Verification items for the finished model (mm, model axes). Coordinates: 2 decimals unless noted, no trailing zeros. Loops run counter-clockwise (first coordinate to the right, second up) from the corner with the lowest first, then second, coordinate; pieces in that order, holes last. Notation, with made-up numbers: M 28.5,-27.5 L 44.5,-27.5 A35 cw 44.5,8.5 Z; hole C 66.25,3 d8. An arc over 180 degrees is marked long. Write item = value, one per line. Start each with the question number.
```python
from build123d import *

# Parameters (mm, degrees)
ESBO_O1_R                = 1.65
RESSALTO_EXTRUS_O1_DEPTH = 3
FILETE1_R                = 8


with BuildPart() as part:
    # Esboço1 → Ressalto-extrusão1 (new body)
    with BuildSketch(Plane.XY):
        with BuildLine():
            Line((-5.233177242, 16.48), (-11.2845681, 3.348148148))
            ThreePointArc((-11.2845681, 3.348148148), (-11.621333239, 2.490590121), (-11.85726917, 1.6))
            Line((-11.85726917, 1.6), (-7.48080878, 1.6))
            ThreePointArc((-7.48080878, 1.6), (0, 7.65), (7.48080878, 1.6))
            Line((7.48080878, 1.6), (11.85726917, 1.6))
            ThreePointArc((11.85726917, 1.6), (11.621333239, 2.490590121), (11.2845681, 3.348148148))
            Line((11.2845681, 3.348148148), (5.233177242, 16.48))
            Line((5.233177242, 16.48), (-5.233177242, 16.48))
        make_face()
        with Locations((0, 13.5)):
            Circle(ESBO_O1_R, mode=Mode.SUBTRACT)
    extrude(amount=RESSALTO_EXTRUS_O1_DEPTH)

    # Filete1
    filete1_edges = [part.edges().sort_by_distance(p)[0] for p in [
        (-5.233177242, 16.48, 1.5),
        (5.233177242, 16.48, 1.5),
    ]]
    fillet(filete1_edges, radius=FILETE1_R)


solid = part.part
```
Q1. Sectioned sample at D-D on x = -10.25. Record the cut outline in (y, z), plus the area to 3 significant figures.
Q2. Sectioned sample at A-A on y = 13. Record the cut outline in (x, z).
Q3. Sectioned sample at B-B on z = 1.2. Record the cut outline in (x, y), plus the area to 3 significant figures.
Q4. Gauge pin test, flat end, axial feed: pin 1 (1 mm diameter, centred on y = 10, z = 1, fed in from -X). Record the tip position at first contact, or that the pin passes through.
Q5. Mould release check, pull along X, two halves, no side actions. Record for faces 1 (the face through (0, 9, 3)), 2 (the face through (-0.15, 7.65, 1.48)), 3 (the face through (-11.62, 2.5, 1.48)): +X half, -X half, draft (parallel to the pull), parting line (faces both ways), or undercut.
Q6. Scan lines: L1, parallel to Y at x = 0, z = 1.15; L2, parallel to X at y = 5.25, z = 1.35; L3, parallel to X at y = 12.75, z = 1.1. Record each from-to range of solid material in increasing order. Write a range as [from, to].
Q7. Sectioned sample at C-C on y = 6.25. Record the cut outline in (x, z), plus the area to 3 significant figures.
Solutions:
q1.outline = M 1.6,0 L 5.59,0 L 5.59,3 L 1.6,3 Z
q1.area = 12.0 mm²
q2.outline = M -6.71,0 L -1.57,0 L -1.57,3 L -6.71,3 Z; M 1.57,0 L 6.71,0 L 6.71,3 L 1.57,3 Z
q3.outline = M -11.86,1.6 L -7.48,1.6 A7.65 cw 7.48,1.6 L 11.86,1.6 A8 ccw 11.28,3.35 L 7.38,11.83 A8 ccw 0.11,16.48 L -0.11,16.48 A8 ccw -7.38,11.83 L -11.28,3.35 A8 ccw Z; hole C 0,13.5 d3.3
q3.area = 172 mm²
q4.pin_1 = -8.45
q5.face_1 = draft
q5.face_2 = undercut
q5.face_3 = -X half
q6.L1 = [7.65, 11.85], [15.15, 16.48]
q6.L2 = [-10.41, -5.56], [5.56, 10.41]
q6.L3 = [-6.88, -1.47], [1.47, 6.88]
q7.outline = M -9.95,0 L -4.41,0 L -4.41,3 L -9.95,3 Z; M 4.41,0 L 9.95,0 L 9.95,3 L 4.41,3 Z
q7.area = 33.2 mm²
